```python
from build123d import *

# Parameters (mm, degrees)
F1_DEPTH = 63.5
F2_DEPTH = 25.4
F3_DEPTH = 7.9375
F0_W     = 25.4
F0_H     = 28.575
F5_R     = 6.35


with BuildPart() as f1:
    # F0 (on Front) → F1 (new body, symmetric)
    with BuildSketch(Plane.XZ):
        Polygon((-41.275, 9.525), (-41.275, -9.525), (41.275, -9.525), (41.275, 9.525), (22.225, 9.525), align=None)
    extrude(amount=F1_DEPTH, both=True)

    # F0 (on Front) → F2 (join, symmetric)
    with BuildSketch(Plane.XZ):
        with BuildLine():
            Line((22.225, 9.525), (41.275, 9.525))
            Line((41.275, 9.525), (41.275, 27.0002))
            ThreePointArc((41.275, 27.0002), (45.92468, 38.22552), (57.15, 42.8752))
            Line((57.15, 42.8752), (60.325, 42.8752))
            Line((60.325, 42.8752), (60.325, 61.9252))
            Line((60.325, 61.9252), (57.15, 61.9252))
            ThreePointArc((57.15, 61.9252), (32.454296, 51.695904), (22.225, 27.0002))
            Line((22.225, 27.0002), (22.225, 9.525))
        make_face()
        Polygon((60.325, 66.675), (60.325, 61.9252), (60.325, 42.8752), (60.325, 38.1), (85.725, 38.1), (85.725, 66.675), align=None)
    extrude(amount=F2_DEPTH, both=True)

    # F0 (on Front) → F3 (join, symmetric)
    with BuildSketch(Plane.XZ):
        with BuildLine():
            add(Edge.make_bspline(
                [(-41.275, 9.525), (-28.23109, 40.560842), (8.36162, 79.393923), (57.15, 61.9252)],
                knots=[0, 0, 0, 0, 111.504536, 111.504536, 111.504536, 111.504536], degree=3))
            Line((-41.275, 9.525), (22.225, 9.525))
            Line((22.225, 9.525), (22.225, 27.0002))
            ThreePointArc((22.225, 27.0002), (32.454296, 51.695904), (57.15, 61.9252))
        make_face()
    extrude(amount=F3_DEPTH, both=True)

    # F0 (on Front) → F4 (revolve)
    with BuildSketch(Plane.XZ):
        with Locations((98.425, 52.3875)):
            Rectangle(F0_W, F0_H)
    revolve(axis=Axis((85.725, 0, 52.3875), (0, 0, 1)))

    # F5
    f5_edges = [f1.edges().sort_by_distance(p)[0] for p in [
        (-41.275, -63.5, 0),
        (41.275, -63.5, 0),
        (41.275, 63.5, 0),
        (-41.275, 63.5, 0),
    ]]
    fillet(f5_edges, radius=F5_R)


solid = f1.part
```
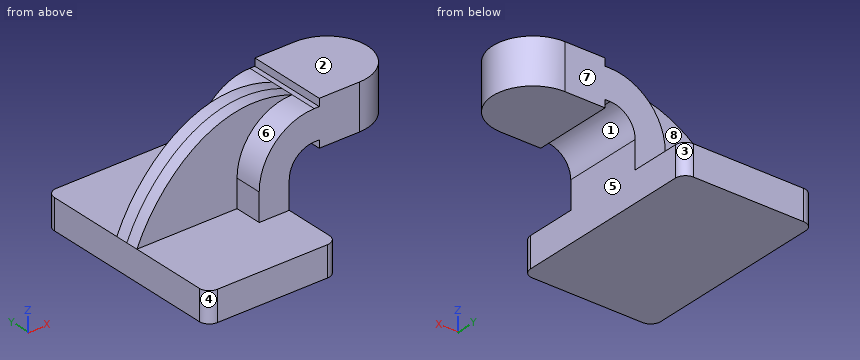
The listing builds one solid part. Answer for the finished solid, in the listing's coordinates (mm). Face numbers are marked on the shaded views. A direction names the side the tool comes from. Coordinates: 2 decimals unless noted, no trailing zeros. Write each loop counter-clockwise with the first axis right and the second up, starting at its lowest first coordinate (ties: lowest second). Pieces come first, ordered by that corner, then holes. Notation, with made-up numbers: (69.5, 19.25) - (125.5, 19.25) arc R20 ccw to (125.5, 39.25) - close; hole circle Ø10 at (78.5, -8.5). An arc over 180 degrees is marked (long way). Return JSON: item names as keys, results as strings. Group by question number.
1. Which of the six approach directions +Z, -Z, +X, -X, +Y, -Y give full straight-line access (tool end or side, diameter ignored) to the marked faces 5, 6, 7 and 8?
2. Given pin 1 (6 mm diameter, centred on x = 86.5, z = 38, fed in from +Y); pin 2 (3.5 mm diameter, centred on x = 58, y = -6.5, fed in from -Z); pin 3 (1.6 mm diameter, centred on x = 58.5, y = 4, fed in from +Z), each flat-ended and moving along its own axis, determine where each tip first touches the part or whether it passes through.
3. Determine the mould class of the marked faces 1, 2, 3 and 4 for opening direction X: released by +X, released by -X, zero draft, split by the parting line, or undercut.
4. Straight lines are drawn through the part: L1, parallel to X at y = 13.5, z = 26 (3 decimals); L2, parallel to Y at x = 15, z = 48.5; L3, parallel to Z at x = -6, y = -17.5 (3 decimals). For each, find the intervals that lie inside material, in ascending order.
5. A cutting plane is placed at B-B, the plane y = 29. Determine the outline of the cut face in (x, z) (3 decimals), plus the area to 3 significant figures.
6. A cutting plane is placed at A-A, the plane z = -5. Determine the outline of the cut face in (x, y) (3 decimals), plus the area to 3 significant figures.
Ans:
{
 "1": {"face 5": "-Z, +X, +Y, -Y", "face 6": "+Z, -X, -Y", "face 7": "+Z, +X, -X, +Y", "face 8": "+Z, -X, +Y"},
 "2": {"pin 1": "y = 25.4", "pin 2": "z = 42.85", "pin 3": "z = 61.93"},
 "3": {"face 1": "undercut", "face 2": "zero draft", "face 3": "released by +X", "face 4": "released by -X"},
 "4": {"L1": "22.225 to 41.275", "L2": "-7.94 to 7.94", "L3": "-9.525 to 9.525"},
 "5": {"outline": "(-41.275, -9.525) - (41.275, -9.525) - (41.275, 9.525) - (-41.275, 9.525) - close", "area": "1,570 mm²"},
 "6": {"outline": "(-41.275, -57.15) arc R6.35 ccw to (-34.925, -63.5) - (34.925, -63.5) arc R6.35 ccw to (41.275, -57.15) - (41.275, 57.15) arc R6.35 ccw to (34.925, 63.5) - (-34.925, 63.5) arc R6.35 ccw to (-41.275, 57.15) - close", "area": "10,400 mm²"}
}
